```python
from build123d import *

# Parameters (mm, degrees)
AUFSATZ_LINEAR_AUSTRAGEN1_DEPTH             = 150
AUFSATZ_LINEAR_AUSTRAGEN2_REACH             = 712.634
AUFSATZ_LINEAR_AUSTRAGEN2_DIRECTION_2_REACH = 712.634


with BuildPart() as part:
    # Skizze1 → Aufsatz-Linear austragen1 (new, symmetric)
    with BuildSketch(Plane.XY):
        Polygon((0, 0), (-202.072594216, 350), (397.927405784, 350), (397.927405784, 0), align=None)
    extrude(amount=AUFSATZ_LINEAR_AUSTRAGEN1_DEPTH, both=True)

    # Aufsatz-Linear austragen2: up to this face of the body (flat: up to its plane)
    aufsatz_linear_austragen2_end = Plane(part.part.faces().sort_by_distance((198.963702892, 0, 0))[0])
    # Skizze3 → Aufsatz-Linear austragen2 (add, up to the picked face)
    with BuildSketch(Plane(origin=(-202.072594216, 350, 0), x_dir=(0, 0, -1), z_dir=(-0.4999999999999981, 0.8660254037844398, 0)), mode=Mode.PRIVATE) as aufsatz_linear_austragen2_sk1:
        with BuildLine():
            Line((150, 0), (-150, 0))
            ThreePointArc((-150, 0), (0, 150), (150, 0))
        make_face()
    aufsatz_linear_austragen2_tool1 = split(extrude(aufsatz_linear_austragen2_sk1.sketch, amount=-AUFSATZ_LINEAR_AUSTRAGEN2_REACH, mode=Mode.PRIVATE), bisect_by=aufsatz_linear_austragen2_end, keep=Keep.BOTH, mode=Mode.PRIVATE)
    add(aufsatz_linear_austragen2_tool1.solids().sort_by(Axis((-257.205484, 318.169011, 0), (0.4999999999999981, -0.8660254037844398, 0)))[0])

    # Aufsatz-Linear austragen2 direction 2: up to this face of the body (flat: up to its plane)
    aufsatz_linear_austragen2_direction_2_end = Plane(part.part.faces().sort_by_distance((97.927405784, 350, 0))[0])
    # Skizze3 → Aufsatz-Linear austragen2 direction 2 (add, up to the picked face)
    with BuildSketch(Plane(origin=(-202.072594216, 350, 0), x_dir=(0, 0, -1), z_dir=(-0.4999999999999981, 0.8660254037844398, 0)), mode=Mode.PRIVATE) as aufsatz_linear_austragen2_direction_2_sk1:
        with BuildLine():
            Line((150, 0), (-150, 0))
            ThreePointArc((-150, 0), (0, 150), (150, 0))
        make_face()
    aufsatz_linear_austragen2_direction_2_tool1 = split(extrude(aufsatz_linear_austragen2_direction_2_sk1.sketch, amount=AUFSATZ_LINEAR_AUSTRAGEN2_DIRECTION_2_REACH, mode=Mode.PRIVATE), bisect_by=aufsatz_linear_austragen2_direction_2_end, keep=Keep.BOTH, mode=Mode.PRIVATE)
    add(aufsatz_linear_austragen2_direction_2_tool1.solids().sort_by(Axis((-257.205484, 318.169011, 0), (-0.4999999999999981, 0.8660254037844398, 0)))[0])


solid = part.part
```
The model under review builds one solid part; all positions refer to its coordinate system, in mm. Give positions to 0.01 mm unless a question says otherwise; leave off trailing zeros. Write each loop counter-clockwise with the first axis right and the second up, starting at its lowest first coordinate (ties: lowest second). Pieces come first, ordered by that corner, then holes. Notation, with made-up numbers: M 32,37.5 L 86,37.5 A16 ccw 86,63.5 Z; hole C 18.25,55.25 d2. An arc over 180 degrees is marked long. Write item = value, one per line. Start each with the question number.
Q1. We need section A-A (z = 57). State the section outline as (x, y) points.
Q2. Clearance check with flat-ended pins moving along their axes: pin 1 (1 mm diameter, centred on x = -282, y = 213.5, fed in from -Z); pin 2 (5 mm diameter, centred on x = -206, z = -101, fed in from -Y); pin 3 (3 mm diameter, centred on y = 295, z = 74.5, fed in from -X). State where each tip first meets the part, or that it passes through.
Q3. We need section B-B (z = -42.5). State the section outline as (x, y) points.
Q4. For line 1 (Y direction, x = -169, z = -78); line 2 (X direction, y = 29.5, z = 81.5); line 3 (X direction, y = 234.5, z = -70.5), list the stretches that pass through material, from the lowest coordinate up.
Result set:
q1.outline = M -362.28,350 L -160.21,0 L 397.93,0 L 397.93,350 Z
q2.pin_1 = -61.15
q2.pin_2 = 128.77
q2.pin_3 = -321.96
q3.outline = M -368.18,350 L -166.11,0 L 397.93,0 L 397.93,350 Z
q4.line_1 = 36.47 to 350
q4.line_2 = -162.44 to 397.93
q4.line_3 = -288.27 to 397.93
